Drawing for the job (mm, zero at the part's lowest x, y, z). A direction names the side the tool comes from. Give positions to 0.01 mm unless a question says otherwise; leave off trailing zeros. Loops run counter-clockwise (first coordinate to the right, second up) from the corner with the lowest first, then second, coordinate; pieces in that order, holes last.
1) Band-saw the part on B-B on x = 37. List the corners of the cut face in (y, z).
2) Wall check: line 1 (Z direction, x = 13.5, y = 3.5); line 2 (Y direction, x = 36.5, z = 18.25); line 3 (Y direction, x = 5, z = 27). Give the ranges that are in metal, low to high.
3) Band-saw the part on A-A on z = 23.25. List the corners of the cut face in (x, y), then the cut area to 3 significant figures.
4) Band-saw the part on C-C on y = 3.5. List the corners of the cut face in (x, z).
5) Band-saw the part on D-D on x = 14.5. List the corners of the cut face in (y, z), then the cut area to 3 significant figures.
6) 3-axis set-ups, long thin cutter, end or side, ignore diameter. For the marked faces 1, 2 and 3: which of +Z, -Z, +X, -X, +Y, -Y reach the whole face in a straight line?
7) Flat gauge pins, fed straight in: P1, Ø4.5, axis at x = 15.5, z = 19.5, coming from the -Y side; P2, Ø1, axis at x = 31, y = 6, coming from the +Z side; P3, Ø5, axis at x = 37.5, z = 20.5, coming from the -Y side. Where does each tip first touch, or does it go through?
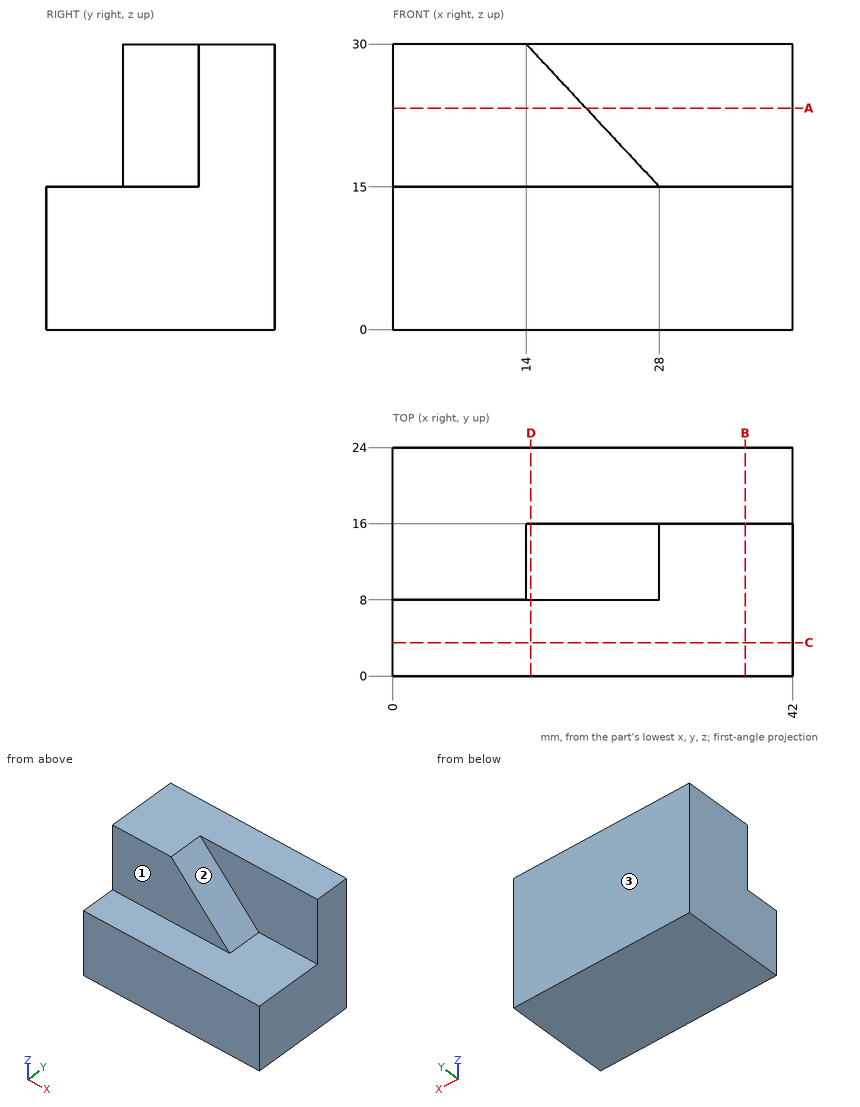
Findings below:
1. outline: (0, 0) - (24, 0) - (24, 30) - (16, 30) - (16, 15) - (0, 15) - close
2. line 1: z = 0 to 15
2. line 2: y = 16 to 24
2. line 3: y = 8 to 24
3. outline: (0, 8) - (20.3, 8) - (20.3, 16) - (42, 16) - (42, 24) - (0, 24) - close
3. area: 498 mm2
4. outline: (0, 0) - (42, 0) - (42, 15) - (0, 15) - close
5. outline: (0, 0) - (24, 0) - (24, 30) - (16, 30) - (16, 29.46) - (8, 29.46) - (8, 15) - (0, 15) - close
5. area: 596 mm2
6. face 1: +Z, +X, -X, -Y
6. face 2: +Z, +X, -Y
6. face 3: +Z, -Z, +X, -X, +Y
7. P1: stops at y = 8
7. P2: stops at z = 15
7. P3: stops at y = 16
